from build123d import *

# Parameters (mm, degrees)
SKETCH1_R           = 2.5
BOSS_EXTRUDE1_DEPTH = 300


with BuildPart() as part:
    # Sketch1 → Boss-Extrude1 (new body)
    with BuildSketch(Plane(origin=(0, 0, 0), x_dir=(-1, 0, 0), z_dir=(0, 0, -1))):
        with BuildLine():
            Line((-20, 19), (-20, 13.2))
            Line((-20, 13.2), (-18.2, 13.2))
            Line((-18.2, 13.2), (-18.2, 14.95))
            ThreePointArc((-18.2, 14.95), (-18.053553391, 15.303553391), (-17.7, 15.45))
            Line((-17.7, 15.45), (-16.607106781, 15.45))
            ThreePointArc((-16.607106781, 15.45), (-16.415765065, 15.411939766), (-16.253553391, 15.303553391))
            Line((-16.253553391, 15.303553391), (-14.046446609, 13.096446609))
            ThreePointArc((-14.046446609, 13.096446609), (-13.938060234, 12.934234935), (-13.9, 12.742893219))
            Line((-13.9, 12.742893219), (-13.9, 7.257106781))
            ThreePointArc((-13.9, 7.257106781), (-13.938060234, 7.065765065), (-14.046446609, 6.903553391))
            Line((-14.046446609, 6.903553391), (-16.253553391, 4.696446609))
            ThreePointArc((-16.253553391, 4.696446609), (-16.415765065, 4.588060234), (-16.607106781, 4.55))
            Line((-16.607106781, 4.55), (-17.7, 4.55))
            ThreePointArc((-17.7, 4.55), (-18.053553391, 4.696446609), (-18.2, 5.05))
            Line((-18.2, 5.05), (-18.2, 6.8))
            Line((-18.2, 6.8), (-20, 6.8))
            Line((-20, 6.8), (-20, 1))
            ThreePointArc((-20, 1), (-19.707106781, 0.292893219), (-19, 0))
            Line((-19, 0), (-13.2, 0))
            Line((-13.2, 0), (-13.2, 1.8))
            Line((-13.2, 1.8), (-14.95, 1.8))
            ThreePointArc((-14.95, 1.8), (-15.303553391, 1.946446609), (-15.45, 2.3))
            Line((-15.45, 2.3), (-15.45, 3.392893219))
            ThreePointArc((-15.45, 3.392893219), (-15.411939766, 3.584234935), (-15.303553391, 3.746446609))
            Line((-15.303553391, 3.746446609), (-13.096446609, 5.953553391))
            ThreePointArc((-13.096446609, 5.953553391), (-12.934234935, 6.061939766), (-12.742893219, 6.1))
            Line((-12.742893219, 6.1), (-7.257106781, 6.1))
            ThreePointArc((-7.257106781, 6.1), (-7.065765065, 6.061939766), (-6.903553391, 5.953553391))
            Line((-6.903553391, 5.953553391), (-4.696446609, 3.746446609))
            ThreePointArc((-4.696446609, 3.746446609), (-4.588060234, 3.584234935), (-4.55, 3.392893219))
            Line((-4.55, 3.392893219), (-4.55, 2.3))
            ThreePointArc((-4.55, 2.3), (-4.696446609, 1.946446609), (-5.05, 1.8))
            Line((-5.05, 1.8), (-6.8, 1.8))
            Line((-6.8, 1.8), (-6.8, 0))
            Line((-6.8, 0), (-1, 0))
            ThreePointArc((-1, 0), (-0.292893219, 0.292893219), (0, 1))
            Line((0, 1), (0, 6.8))
            Line((0, 6.8), (-1.8, 6.8))
            Line((-1.8, 6.8), (-1.8, 5.05))
            ThreePointArc((-1.8, 5.05), (-1.946446609, 4.696446609), (-2.3, 4.55))
            Line((-2.3, 4.55), (-3.392893219, 4.55))
            ThreePointArc((-3.392893219, 4.55), (-3.584234935, 4.588060234), (-3.746446609, 4.696446609))
            Line((-3.746446609, 4.696446609), (-5.953553391, 6.903553391))
            ThreePointArc((-5.953553391, 6.903553391), (-6.061939766, 7.065765065), (-6.1, 7.257106781))
            Line((-6.1, 7.257106781), (-6.1, 12.742893219))
            ThreePointArc((-6.1, 12.742893219), (-6.061939766, 12.934234935), (-5.953553391, 13.096446609))
            Line((-5.953553391, 13.096446609), (-3.746446609, 15.303553391))
            ThreePointArc((-3.746446609, 15.303553391), (-3.584234935, 15.411939766), (-3.392893219, 15.45))
            Line((-3.392893219, 15.45), (-2.3, 15.45))
            ThreePointArc((-2.3, 15.45), (-1.946446609, 15.303553391), (-1.8, 14.95))
            Line((-1.8, 14.95), (-1.8, 13.2))
            Line((-1.8, 13.2), (0, 13.2))
            Line((0, 13.2), (0, 19))
            ThreePointArc((0, 19), (-0.292893219, 19.707106781), (-1, 20))
            Line((-1, 20), (-6.8, 20))
            Line((-6.8, 20), (-6.8, 18.2))
            Line((-6.8, 18.2), (-5.05, 18.2))
            ThreePointArc((-5.05, 18.2), (-4.696446609, 18.053553391), (-4.55, 17.7))
            Line((-4.55, 17.7), (-4.55, 16.607106781))
            ThreePointArc((-4.55, 16.607106781), (-4.588060234, 16.415765065), (-4.696446609, 16.253553391))
            Line((-4.696446609, 16.253553391), (-6.903553391, 14.046446609))
            ThreePointArc((-6.903553391, 14.046446609), (-7.065765065, 13.938060234), (-7.257106781, 13.9))
            Line((-7.257106781, 13.9), (-12.742893219, 13.9))
            ThreePointArc((-12.742893219, 13.9), (-12.934234935, 13.938060234), (-13.096446609, 14.046446609))
            Line((-13.096446609, 14.046446609), (-15.303553391, 16.253553391))
            ThreePointArc((-15.303553391, 16.253553391), (-15.411939766, 16.415765065), (-15.45, 16.607106781))
            Line((-15.45, 16.607106781), (-15.45, 17.7))
            ThreePointArc((-15.45, 17.7), (-15.303553391, 18.053553391), (-14.95, 18.2))
            Line((-14.95, 18.2), (-13.2, 18.2))
            Line((-13.2, 18.2), (-13.2, 20))
            Line((-13.2, 20), (-19, 20))
            ThreePointArc((-19, 20), (-19.707106781, 19.707106781), (-20, 19))
        make_face()
        with Locations((-10, 10)):
            Circle(SKETCH1_R, mode=Mode.SUBTRACT)
    extrude(amount=-BOSS_EXTRUDE1_DEPTH)


solid = part.part
For this review, take the finished solid that the model builds, in its own axes (mm). A direction names the side the tool comes from. Round coordinates to 2 decimals unless told otherwise and drop trailing zeros. Write each loop counter-clockwise with the first axis right and the second up, starting at its lowest first coordinate (ties: lowest second). Pieces come first, ordered by that corner, then holes. Notation, with made-up numbers: (52.5, 58) - (102.5, 58) arc R22 ccw to (102.5, 96) - close; hole circle Ø7 at (23, 41.5). An arc over 180 degrees is marked (long way). Use a Markdown table: item, result.
Q1. We need section A-A (x = 10). Give the boundary of the cut face in (y, z).
Derived:
| item | result |
|---|---|
| outline | (6.1, 0) - (7.5, 0) - (7.5, 300) - (6.1, 300) - close; (12.5, 0) - (13.9, 0) - (13.9, 300) - (12.5, 300) - close |
Q2. Wall thickness on line 1 along Y through (x, z) = (1.25, 181); line 2 along X through (y, z) = (14.5, 156); line 3 along Y through (x, z) = (15, 252): over which ranges is each line inside the solid? List them lowest first.
Derived:
| item | result |
|---|---|
| line 1 | y = 0 to 6.8, 13.2 to 20 |
| line 2 | x = 0 to 1.8, 4.55 to 6.45, 13.55 to 15.45, 18.2 to 20 |
| line 3 | y = 0 to 1.8, 4.05 to 5.95, 14.05 to 15.95, 18.2 to 20 |
Q3. Machinability: for faces 1 (the flat face through (6.1, 10, 148)), 2 (the flat face through (10, 13.9, 148)), 3 (the cylindrical face through (10.54, 7.56, 147.9)), 4 (the flat face through (13.9, 10, 148)), 5 (the flat face through (12, 12, 0)), which of the approach directions +Z, -Z, +X, -X, +Y, -Y give a long, thin tool a straight path to every point of the face, cutting with its end or side? Answer none if there is none.
Derived:
| item | result |
|---|---|
| face 1 | +Z, -Z, -X |
| face 2 | +Z, -Z, +Y |
| face 3 | +Z, -Z |
| face 4 | +Z, -Z, +X |
| face 5 | -Z, +X, -X, +Y, -Y |
Q4. Clearance check with a flat-ended pin moving along its axis: pin 1 (1 mm diameter, centred on y = 11.5, z = 44.5, fed in from -X). State where the tip first meets the part, or that it passes through.
Derived:
| item | result |
|---|---|
| pin 1 | stops at x = 6.1 |
Q5. The part is to be moulded in two halves that separate along X. For faces 6 (the flat face through (20, 16, 148)), 7 (the flat face through (4, 0, 148)), 8 (the flat face through (10, 6.1, 148)), say which applies: pulls with the +X half, pulls with the -X half, needs draft (parallel to the pull), parting line crosses it, or undercut.
Derived:
| item | result |
|---|---|
| face 6 | pulls with the +X half |
| face 7 | needs draft |
| face 8 | undercut |
